Read the model definition and answer for the solid it produces. Units are mm, in the model's axes. Face numbers are marked on the shaded views. A direction names the side the tool comes from. Coordinates: 2 decimals unless noted, no trailing zeros. Loops run counter-clockwise (first coordinate to the right, second up) from the corner with the lowest first, then second, coordinate; pieces in that order, holes last. Notation, with made-up numbers: (53, -5) - (110, -5) arc R30 cw to (110, 22) - close; hole circle Ø1 at (78, -28.75). An arc over 180 degrees is marked (long way). Use one line per item in the form item = value. Start each with the question number.
1) The mould has two halves that part along X. Classify the marked faces 1, 2 and 3: released by +X, released by -X, zero draft, split by the parting line, or undercut.
2) Consider line 1 (X direction, y = 6, z = -0.4); line 2 (X direction, y = 5.5, z = -0.2); line 3 (Y direction, x = -5.5, z = 0.05). Determine where each line is inside the solid, lowest interval first.
3) A cutting plane is placed at A-A (z = 0.2). Give the vertices of the cut face in (x, y).
4) A cutting plane is placed at D-D (x = 0). Give the vertices of the cut face in (y, z).
5) Which of the six approach directions +Z, -Z, +X, -X, +Y, -Y give full straight-line access (tool end or side, diameter ignored) to the marked faces 4 and 5?
6) A cutting plane is placed at C-C (x = 6.5). Give the vertices of the cut face in (y, z), and give its area (3 significant figures).
7) A cutting plane is placed at B-B (y = 0.5). Give the vertices of the cut face in (x, z).
from build123d import *

# Parameters (mm, degrees)
SKETCH3_W               = 8.382
SKETCH3_H               = 0.889
CUT_EXTRUDE1_DEPTH      = 1.4445
CUT_EXTRUDE1_DEPTH_BACK = 1.4445
FILLET1_R               = 1.00584
FILLET2_R               = 0.653796
FILLET3_R               = 0.22225


with BuildPart() as part:
    # Sketch3 → Revolve1 (revolve)
    with BuildSketch(Plane(origin=(0, 0, 0), x_dir=(1, 0, 0), z_dir=(0, 1, 0))):
        with Locations((-4.191, 0)):
            Rectangle(SKETCH3_W, SKETCH3_H)
    revolve(axis=Axis((0, 0, -0.4445), (0, 0, 1)))

    # Sketch4 → Cut-Extrude1 (cut, two sides)
    with BuildSketch(Plane.XY) as cut_extrude1_sk:
        with BuildLine():
            Line((1.043411472, 3.664340664), (1.907952406, 6.700508642))
            ThreePointArc((1.907952406, 6.700508642), (5.560104779, 4.197896295), (6.966857143, 0))
            Line((6.966857143, 0), (3.81, 0))
            ThreePointArc((3.81, 0), (3.664340664, -1.043411472), (3.2385, -2.00704204))
            Line((3.2385, -2.00704204), (4.167000213, -7.27282842))
            ThreePointArc((4.167000213, -7.27282842), (0, -8.382), (-4.167000213, -7.27282842))
            Line((-4.167000213, -7.27282842), (-3.2385, -2.00704204))
            ThreePointArc((-3.2385, -2.00704204), (-3.664340664, -1.043411472), (-3.81, 0))
            Line((-3.81, 0), (-6.966857143, 0))
            ThreePointArc((-6.966857143, 0), (-5.560104779, 4.197896295), (-1.907952406, 6.700508642))
            Line((-1.907952406, 6.700508642), (-1.043411472, 3.664340664))
            ThreePointArc((-1.043411472, 3.664340664), (0, 3.81), (1.043411472, 3.664340664))
        make_face()
    extrude(amount=CUT_EXTRUDE1_DEPTH, mode=Mode.SUBTRACT)
    extrude(cut_extrude1_sk.sketch, amount=-CUT_EXTRUDE1_DEPTH_BACK, mode=Mode.SUBTRACT)

    # Fillet1
    fillet1_edges = [part.edges().sort_by_distance(p)[0] for p in [
        (1.907952406, 6.700508642, 0),
        (6.966857143, 0, 0),
        (-6.966857143, 0, 0),
        (-1.907952406, 6.700508642, 0),
    ]]
    fillet(fillet1_edges, radius=FILLET1_R)

    # Fillet2
    fillet2_edges = [part.edges().sort_by_distance(p)[0] for p in [
        (4.167000213, -7.27282842, 0),
        (-4.167000213, -7.27282842, 0),
    ]]
    fillet(fillet2_edges, radius=FILLET2_R)

    # Fillet3
    fillet3_edges = [part.edges().sort_by_distance(p)[0] for p in [
        (-1.043411472, 3.664340664, 0),
        (1.043411472, 3.664340664, 0),
        (3.81, 0, 0),
        (3.2385, -2.00704204, 0),
        (-3.2385, -2.00704204, 0),
        (-3.81, 0, 0),
    ]]
    fillet(fillet3_edges, radius=FILLET3_R)


solid = part.part
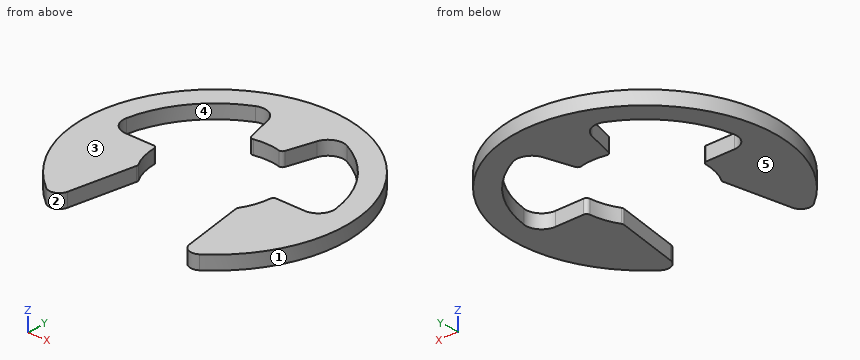
Found:
q1.face_1 = split by the parting line
q1.face_2 = undercut
q1.face_3 = zero draft
q2.line_1 = -5.85 to -3.54, -1.79 to 1.79, 3.54 to 5.85
q2.line_2 = -6.33 to -4.28, -1.57 to 1.57, 4.28 to 6.33
q2.line_3 = -6.33 to 0, 4.28 to 6.33
q3.outline = (-6.87, 1.18) arc R6.97 cw to (-3.01, 6.28) arc R1.01 cw to (-1.61, 5.65) - (-1.1, 3.87) arc R0.22 ccw to (-0.84, 3.72) arc R3.81 cw to (0.84, 3.72) arc R0.22 ccw to (1.1, 3.87) - (1.61, 5.65) arc R1.01 cw to (3.01, 6.28) arc R6.97 cw to (6.87, 1.18) arc R1.01 cw to (5.88, 0) - (4.03, 0) arc R0.22 ccw to (3.8, -0.21) arc R3.81 cw to (3.28, -1.94) arc R0.22 ccw to (3.25, -2.09) - (3.99, -6.29) arc R0.65 ccw to (5.03, -6.7) arc R8.38 ccw (long way) to (-5.03, -6.7) arc R0.65 ccw to (-3.99, -6.29) - (-3.25, -2.09) arc R0.22 ccw to (-3.28, -1.94) arc R3.81 cw to (-3.8, -0.21) arc R0.22 ccw to (-4.03, 0) - (-5.88, 0) arc R1.01 cw to start
q4.outline = (3.81, -0.44) - (8.38, -0.44) - (8.38, 0.44) - (3.81, 0.44) - close
q5.face_4 = +Z, -Z
q5.face_5 = -Z, +X, -X, +Y, -Y
q6.outline = (-5.29, -0.44) - (0.22, -0.44) - (0.22, 0.44) - (-5.29, 0.44) - close; (2.51, -0.44) - (5.29, -0.44) - (5.29, 0.44) - (2.51, 0.44) - close
q6.area = 7.37 mm^2
q7.outline = (-8.37, -0.44) - (-6.74, -0.44) - (-6.74, 0.44) - (-8.37, 0.44) - close; (6.74, -0.44) - (8.37, -0.44) - (8.37, 0.44) - (6.74, 0.44) - close
